The model under review builds one solid part; all positions refer to its coordinate system, in mm. A direction names the side the tool comes from. Give positions to 0.01 mm unless a question says otherwise; leave off trailing zeros. Order: outer loops, then holes, each group sorted by start corner. A loop starts at its lowest first (then second) coordinate and runs counter-clockwise, first axis right, second up. Notation, with made-up numbers: (-18, 73) - (18, 73) arc R33 ccw to (18, 104) - close; hole circle Ø7 at (-16, 53). An arc over 180 degrees is marked (long way). Use CSV: the item, a comma, the result in double quotes.
```python
from build123d import *

# Parameters (mm, degrees)
F0_W     = 19.05
F0_H     = 19.05
F1_DEPTH = 63.5
F3_DEPTH = 19.05


with BuildPart() as f1:
    # F0 (on Front) → F1 (new body)
    with BuildSketch(Plane.XZ):
        with Locations((-21.291444, 24.793022)):
            Rectangle(F0_W, F0_H)
    extrude(amount=F1_DEPTH)

    # F2 (on face) → F3 (join)
    with BuildSketch(Plane.XY.offset(34.318022)):
        Polygon((-30.816444, 0), (-11.766444, 0), (-5.416444, 0), (-5.416444, 31.507518), (-11.766444, 31.507518), (-11.766444, 8.236752), (-30.816444, 8.236752), (-30.816444, 31.507518), (-37.166444, 31.507518), (-37.166444, 0), align=None)
    extrude(amount=-F3_DEPTH)


solid = f1.part
```
Item 1: Clearance check with flat-ended pins moving along their axes: pin 1 (1.9 mm diameter, centred on x = -35, z = 24, fed in from -Y); pin 2 (5.5 mm diameter, centred on y = -18.5, z = 29, fed in from -X); pin 3 (5 mm diameter, centred on x = -32, y = -48.5, fed in from +Z). State where each tip first meets the part, or that it passes through.
Results list:
pin 1,"stops at y = 0"
pin 2,"stops at x = -30.82"
pin 3,"stops at z = 34.32"
Item 2: Take a section at C-C, the plane x = -24.5. Give the boundary of the cut face in (y, z), and give its area (3 significant figures).
Results list:
outline,"(-63.5, 15.27) - (8.24, 15.27) - (8.24, 34.32) - (-63.5, 34.32) - close"
area,"1,370 mm2"
Item 3: Tool access review of faces 4 (the face through (-22, -15, 15.268)), 5 (the face through (-30.816, -31, 25)), 6 (the face through (-21, 8.237, 25)), 7 (the face through (-34, 31.508, 25)), 8 (the face through (-9, 0, 25)): name each direction out of +Z, -Z, +X, -X, +Y, -Y from which nothing blocks a thin tool from reaching the whole face with its end or side.
Results list:
face 4,"-Z, +X, -X, +Y, -Y"
face 5,"+Z, -Z, -X, -Y"
face 6,"+Z, -Z, +Y"
face 7,"+Z, -Z, +X, -X, +Y"
face 8,"+Z, -Z, +X, -Y"
Item 4: Take a section at B-B, the plane y = -15. Give the boundary of the cut face in (x, z), and give its area (3 significant figures).
Results list:
outline,"(-30.82, 15.27) - (-11.77, 15.27) - (-11.77, 34.32) - (-30.82, 34.32) - close"
area,"363 mm2"
Item 5: Take a section at A-A, the plane z = 18.5. Give the boundary of the cut face in (x, y).
Results list:
outline,"(-37.17, 0) - (-30.82, 0) - (-30.82, -63.5) - (-11.77, -63.5) - (-11.77, 0) - (-5.42, 0) - (-5.42, 31.51) - (-11.77, 31.51) - (-11.77, 8.24) - (-30.82, 8.24) - (-30.82, 31.51) - (-37.17, 31.51) - close"
Item 6: Wall thickness on L1, parallel to X at y = 10.5, z = 29; L2, parallel to Y at x = -11, z = 27.5; L3, parallel to Y at x = -30.5, z = 30.75: over which ranges is each line inside the solid? List them lowest first.
Results list:
L1,"x = -37.17 to -30.82, -11.77 to -5.42"
L2,"y = 0 to 31.51"
L3,"y = -63.5 to 8.24"
Item 7: Mouldability with a two-part tool opening along X and no side actions: class faces 1 (the face through (-5.416, 16, 25)), 2 (the face through (-11.766, 20, 25)), 3 (the face through (-34, 0, 25)) as pulls with the +X half, pulls with the -X half, needs draft (parallel to the pull), parting line crosses it, or undercut.
Results list:
face 1,"pulls with the +X half"
face 2,"undercut"
face 3,"needs draft"
